Autodesk Inventor part; units mm, degrees
ref_plane "YZ Plane" through (0, 0, 0) normal (1, 0, 0) x (0, 1, 0)
ref_plane "XZ Plane" through (0, 0, 0) normal (0, 1, 0) x (-1, 0, 0)
ref_plane "XY Plane" through (0, 0, 0) normal (0, 0, 1) x (1, 0, 0)
sketch "Sketch1" plane through (0, 0, 0) normal (0, 1, 0) x (-1, 0, 0)
  circle A0 centre (0, 0) radius 20
  circle A1 centre (0, 0) radius 2.05
  dimension "d0" = 40
  dimension "d1" = 4.1
extrude "Extrusion1" add sketch "Sketch1" along normal blind 2
sketch "Sketch2" plane through (0, 2, 0) normal (0, 1, 0) x (1, 0, 0)
  circle A0 centre (0, 0) radius 18.5
  circle A1 centre (0, 0) radius 2.0967
  circle A2 centre (0, 0) radius 2.05
  dimension "d4" = 37
extrude "Extrusion2" add sketch "Sketch2" along normal blind 0.5 contours A0 | A1
sketch "Sketch3" plane through (0, 2.5, 0) normal (0, 1, 0) x (1, 0, 0)
  circle A0 centre (0, 0) radius 2.05
  circle A1 centre (0, 0) radius 20
extrude "Extrusion3" add sketch "Sketch3" along normal blind 2
fillet "Fillet1" radius 1.5 2 edges at (20, 2, 0) (-20, 2.5, 0)
properties part number "Raket_Hjul"
CAD build for the part. Positions are in the model's coordinates, mm. Round coordinates to 2 decimals unless told otherwise and drop trailing zeros. Loops run counter-clockwise (first coordinate to the right, second up) from the corner with the lowest first, then second, coordinate; pieces in that order, holes last. Notation, with made-up numbers: (22, 34.25) - (63, 34.25) arc R12 ccw to (63, 41.25) - close; hole circle Ø2 at (-10, 6). An arc over 180 degrees is marked (long way). Put each result on its own line as item: value.
1. Two-plate mould, pull along Y, no slides. Class faces 1 (the flat face through (-4, 0, 0)), 2 (the cylindrical face through (-4.336, 4.246, -19.524)), 3 (the cylindrical face through (-4.01, 2.25, -18.06)): released by +Y, released by -Y, zero draft, split by the parting line, or undercut.
Geometry check:
face 1: released by -Y
face 2: zero draft
face 3: undercut
2. Slice it at B-B on y = 1.05. List the corners of the cut face in (x, z).
Geometry check:
outline: circle Ø39.79 at (0, 0); hole circle Ø4.1 at (0, 0)
3. Pin check, flat tips, straight feed: P1, Ø1, axis at y = 3, z = 5.5, coming from the -X side; P2, Ø1.5, axis at y = 0.5, z = 15.5, coming from the -X side. Stop position of each tip, or through.
Geometry check:
P1: x = -19.18
P2: x = -13.51
4. Wall check: line 1 (X direction, y = 3.3, z = 0); line 2 (Z direction, x = -1.5, y = 0.9); line 3 (Z direction, x = 1, y = 3.35). Give the ranges that are in metal, low to high.
Geometry check:
line 1: -19.83 to -2.05, 2.05 to 19.83
line 2: -19.89 to -1.4, 1.4 to 19.89
line 3: -19.83 to -1.79, 1.79 to 19.83
